Drawing for the job (mm, zero at the part's lowest x, y, z). A direction names the side the tool comes from. Round coordinates to 2 decimals unless told otherwise and drop trailing zeros. Write each loop counter-clockwise with the first axis right and the second up, starting at its lowest first coordinate (ties: lowest second). Pieces come first, ordered by that corner, then holes.
Item 1: Band-saw the part on A-A, the plane z = 1.2. Write the cut outline in (x, y).
Item 2: Band-saw the part on C-C, the plane y = 10. Write the cut outline in (x, z).
Item 3: Band-saw the part on B-B, the plane x = 2. Write the cut outline in (y, z).
Item 4: Drop flat-ended pins along their axis: pin 1 Ø3.5 at (x, y) = (3, 3) entering from +Z; pin 2 Ø1.8 at (x, y) = (17, 17) entering from +Z. Give the stop position or say it passes through.
Item 5: Wall check: probe 1 along Y at (x, z) = (3, 0.6); probe 2 along Y at (x, z) = (10, 4.1); probe 3 along Z at (x, y) = (13.75, 1.5). Give the ranges that are in metal, low to high.
Item 6: 3-axis set-ups, long thin cutter, end or side, ignore diameter. For the marked faces 5 and 6: which of +Z, -Z, +X, -X, +Y, -Y reach the whole face in a straight line?
Item 7: Mould opens along Y. For the marked faces 1, 2, 3 and 4 say: +Y half, -Y half, draft (parallel to the pull), parting line (faces both ways), or undercut.
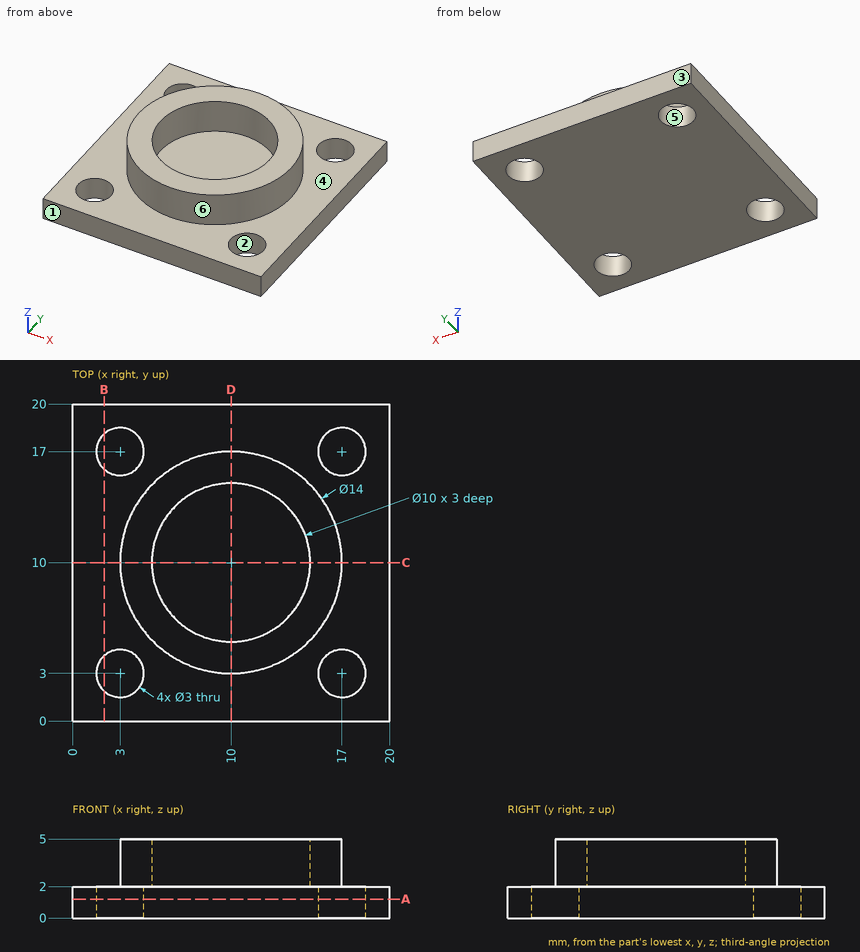
Results:
1. outline: (0, 0) - (20, 0) - (20, 20) - (0, 20) - close; hole circle Ø3 at (3, 3); hole circle Ø3 at (3, 17); hole circle Ø3 at (17, 3); hole circle Ø3 at (17, 17)
2. outline: (0, 0) - (20, 0) - (20, 2) - (17, 2) - (17, 5) - (15, 5) - (15, 2) - (5, 2) - (5, 5) - (3, 5) - (3, 2) - (0, 2) - close
3. outline: (0, 0) - (1.88, 0) - (1.88, 2) - (0, 2) - close; (4.12, 0) - (15.88, 0) - (15.88, 2) - (4.12, 2) - close; (18.12, 0) - (20, 0) - (20, 2) - (18.12, 2) - close
4. pin 1: stops at z = 2
4. pin 2: passes through
5. probe 1: y = 0 to 1.5, 4.5 to 15.5, 18.5 to 20
5. probe 2: y = 3 to 5, 15 to 17
5. probe 3: z = 0 to 2
6. face 5: +Z, -Z
6. face 6: +Z
7. face 1: -Y half
7. face 2: undercut
7. face 3: +Y half
7. face 4: draft
